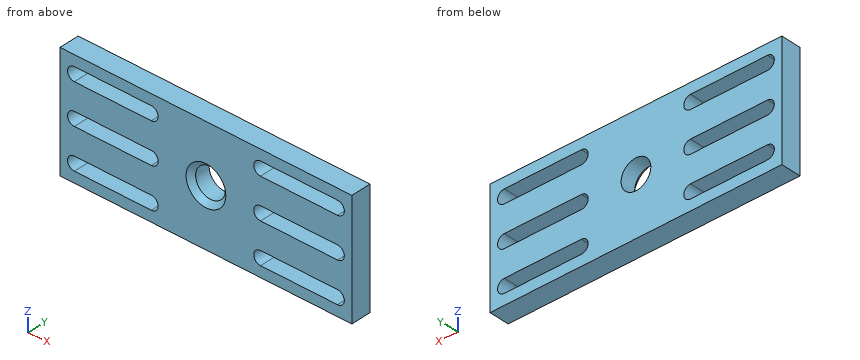
from build123d import *

# Parameters (mm, degrees)
SKETCH1_W           = 290
SKETCH1_H           = 115
BOSS_EXTRUDE1_DEPTH = 20
SKETCH2_R           = 14.75
CUT_EXTRUDE1_DEPTH  = 20
CHAMFER1_SIZE       = 5


with BuildPart() as part:
    # Sketch1 → Boss-Extrude1 (new body)
    with BuildSketch(Plane(origin=(0, 0, 0), x_dir=(1, 0, 0), z_dir=(0, 1, 0))):
        Rectangle(SKETCH1_W, SKETCH1_H)
    extrude(amount=BOSS_EXTRUDE1_DEPTH)

    # Sketch2 → Cut-Extrude1 (cut)
    with BuildSketch(Plane(origin=(0, 20, 0), x_dir=(1, 0, 0), z_dir=(0, 1, 0))):
        Circle(SKETCH2_R)
        with BuildLine():
            Line((-130.75, 6.75), (-54.25, 6.75))
            ThreePointArc((-54.25, 6.75), (-47.5, 0), (-54.25, -6.75))
            Line((-54.25, -6.75), (-130.75, -6.75))
            ThreePointArc((-130.75, -6.75), (-137.5, 0), (-130.75, 6.75))
        make_face()
        with BuildLine():
            Line((-130.75, 46.75), (-54.25, 46.75))
            ThreePointArc((-54.25, 46.75), (-47.5, 40), (-54.25, 33.25))
            Line((-54.25, 33.25), (-130.75, 33.25))
            ThreePointArc((-130.75, 33.25), (-137.5, 40), (-130.75, 46.75))
        make_face()
        with BuildLine():
            Line((-130.75, -33.25), (-54.25, -33.25))
            ThreePointArc((-54.25, -33.25), (-47.5, -40), (-54.25, -46.75))
            Line((-54.25, -46.75), (-130.75, -46.75))
            ThreePointArc((-130.75, -46.75), (-137.5, -40), (-130.75, -33.25))
        make_face()
        with BuildLine():
            Line((54.25, 6.75), (130.75, 6.75))
            ThreePointArc((130.75, 6.75), (137.5, 0), (130.75, -6.75))
            Line((130.75, -6.75), (54.25, -6.75))
            ThreePointArc((54.25, -6.75), (47.5, 0), (54.25, 6.75))
        make_face()
        with BuildLine():
            Line((54.25, -33.25), (130.75, -33.25))
            ThreePointArc((130.75, -33.25), (137.5, -40), (130.75, -46.75))
            Line((130.75, -46.75), (54.25, -46.75))
            ThreePointArc((54.25, -46.75), (47.5, -40), (54.25, -33.25))
        make_face()
        with BuildLine():
            Line((54.25, 46.75), (130.75, 46.75))
            ThreePointArc((130.75, 46.75), (137.5, 40), (130.75, 33.25))
            Line((130.75, 33.25), (54.25, 33.25))
            ThreePointArc((54.25, 33.25), (47.5, 40), (54.25, 46.75))
        make_face()
    extrude(amount=-CUT_EXTRUDE1_DEPTH, mode=Mode.SUBTRACT)

    # Chamfer1
    chamfer1_edges = [part.edges().sort_by_distance(p)[0] for p in [
        (-14.75, 0, 0),
    ]]
    chamfer(chamfer1_edges, length=CHAMFER1_SIZE)


solid = part.part
Model file for the job. Use its own axes, mm. Give positions to 0.01 mm unless a question says otherwise; leave off trailing zeros. Order: outer loops, then holes, each group sorted by start corner. A loop starts at its lowest first (then second) coordinate and runs counter-clockwise, first axis right, second up. Notation, with made-up numbers: (71.5, -5) - (116.5, -5) arc R20 cw to (116.5, -1) - close; hole circle Ø3 at (63, 13.5). An arc over 180 degrees is marked (long way). Write item = value, one per line. Start each with the question number.
1. Cut at D-D, the plane z = -37.5. List the corners of the cut face in (x, y), and give its area (3 significant figures).
2. Cut at B-B, the plane y = 12. State how many separate pieces and enclosed holes the cut face has, and give its area (3 significant figures).
3. Probe line 1 along Z through (x, y) = (89.5, 13.5); line 2 along X through (y, z) = (13.5, 0); line 3 along X through (y, z) = (10.75, -43.5). List the from-to ranges inside material, lowest first.
4. Cut at A-A, the plane z = 0. List the corners of the cut face in (x, y), and give its area (4 significant figures).
5. Cut at C-C, the plane x = -100. List the corners of the cut face in (y, z).
Taken from the geometry:
q1.outline = (-145, 0) - (-137.02, 0) - (-137.02, 20) - (-145, 20) - close; (-47.98, 0) - (47.98, 0) - (47.98, 20) - (-47.98, 20) - close; (137.02, 0) - (145, 0) - (145, 20) - (137.02, 20) - close
q1.area = 2,240 mm²
q2.separate_pieces = 1
q2.enclosed_holes = 7
q2.area = 25,600 mm²
q3.line_1 = -57.5 to -46.75, -33.25 to -6.75, 6.75 to 33.25, 46.75 to 57.5
q3.line_2 = -145 to -137.5, -47.5 to -14.75, 14.75 to 47.5, 137.5 to 145
q3.line_3 = -145 to -136.52, -48.48 to 48.48, 136.52 to 145
q4.outline = (-145, 0) - (-137.5, 0) - (-137.5, 20) - (-145, 20) - close; (-47.5, 0) - (-19.75, 0) - (-14.75, 5) - (-14.75, 20) - (-47.5, 20) - close; (14.75, 5) - (19.75, 0) - (47.5, 0) - (47.5, 20) - (14.75, 20) - close; (137.5, 0) - (145, 0) - (145, 20) - (137.5, 20) - close
q4.area = 1,585 mm²
q5.outline = (0, -57.5) - (20, -57.5) - (20, -46.75) - (0, -46.75) - close; (0, -33.25) - (20, -33.25) - (20, -6.75) - (0, -6.75) - close; (0, 6.75) - (20, 6.75) - (20, 33.25) - (0, 33.25) - close; (0, 46.75) - (20, 46.75) - (20, 57.5) - (0, 57.5) - close
